```python
from build123d import *

# Parameters (mm, degrees)
PAD_DEPTH       = 5
SKETCH001_R     = 1.75
POCKET_DEPTH    = 5.001
SKETCH002_W     = 36.2
SKETCH002_H     = 26.2
POCKET001_DEPTH = 0.5
SKETCH003_R     = 6
POCKET002_DEPTH = 2.8
POCKET003_DEPTH = 2.8
SKETCH005_W     = 6
SKETCH005_H     = 4.5
POCKET004_DEPTH = 5.001
SKETCH006_W     = 14.7
SKETCH006_H     = 3
POCKET005_DEPTH = 5.001
SKETCH007_W     = 35.7
SKETCH007_H     = 18.1
POCKET006_DEPTH = 4.4
SKETCH008_W     = 1.5
SKETCH008_H     = 8
POCKET007_DEPTH = 3.2
POCKET008_DEPTH = 5.001
SKETCH010_W     = 1
SKETCH010_H     = 2
POCKET009_DEPTH = 5.001


with BuildPart() as part:
    # Sketch → Pad (new body)
    with BuildSketch(Plane.XY):
        Polygon((-25, 14.433757), (-25, -14.433757), (0, -28.867513), (25, -14.433757), (25, 14.433757), (0, 28.867513), align=None)
    extrude(amount=PAD_DEPTH)

    # Sketch001 → Pocket (cut, through all)
    with BuildSketch(Plane.XY.offset(5)):
        with Locations((-10.75, -18.619546)):
            Circle(SKETCH001_R)
        with Locations((10.75, 18.619546)):
            Circle(SKETCH001_R)
    extrude(amount=-POCKET_DEPTH, mode=Mode.SUBTRACT)

    # Sketch002 → Pocket001 (cut)
    with BuildSketch(Plane(origin=(0, 0, 0), x_dir=(1, 0, 0), z_dir=(0, 0, -1))):
        with Locations((-5.9, 0.9)):
            Rectangle(SKETCH002_W, SKETCH002_H)
    extrude(amount=-POCKET001_DEPTH, mode=Mode.SUBTRACT)

    # Sketch003 → Pocket002 (cut)
    with BuildSketch(Plane(origin=(0, 0, 0), x_dir=(1, 0, 0), z_dir=(0, 0, -1))):
        with Locations((0, 21)):
            Circle(SKETCH003_R)
    extrude(amount=-POCKET002_DEPTH, mode=Mode.SUBTRACT)

    # Sketch004 → Pocket003 (cut)
    with BuildSketch(Plane(origin=(0, 0, 0), x_dir=(1, 0, 0), z_dir=(0, 0, -1))):
        Polygon((0.841162, 24.139259), (8.085606, 22.198116), (6.403282, 15.919598), (-0.841162, 17.860741), align=None)
    extrude(amount=-POCKET003_DEPTH, mode=Mode.SUBTRACT)

    # Sketch005 → Pocket004 (cut, through all)
    with BuildSketch(Plane(origin=(0, 0, 0), x_dir=(1, 0, 0), z_dir=(0, 0, -1))):
        with Locations((17.35, 7.05)):
            Rectangle(SKETCH005_W, SKETCH005_H)
    extrude(amount=-POCKET004_DEPTH, mode=Mode.SUBTRACT)

    # Sketch006 → Pocket005 (cut, through all)
    with BuildSketch(Plane(origin=(0, 0, 0), x_dir=(1, 0, 0), z_dir=(0, 0, -1))):
        with Locations((0, -22.4)):
            Rectangle(SKETCH006_W, SKETCH006_H)
    extrude(amount=-POCKET005_DEPTH, mode=Mode.SUBTRACT)

    # Sketch007 → Pocket006 (cut)
    with BuildSketch(Plane.XY.offset(5)):
        with Locations((-5.65, 5.383757)):
            Rectangle(SKETCH007_W, SKETCH007_H)
    extrude(amount=-POCKET006_DEPTH, mode=Mode.SUBTRACT)

    # Sketch008 → Pocket007 (cut)
    with BuildSketch(Plane.XY.offset(5)):
        with Locations((-24.25, 5.383757)):
            Rectangle(SKETCH008_W, SKETCH008_H)
    extrude(amount=-POCKET007_DEPTH, mode=Mode.SUBTRACT)

    # Sketch009 → Pocket008 (cut, through all)
    with BuildSketch(Plane(origin=(0, 0, 0), x_dir=(1, 0, 0), z_dir=(0, 0, -1))):
        Polygon((21.1, 3.15), (24.7, 3.15), (24.7, 2), (25.4, 2), (25.4, -2), (24.7, -2), (24.7, -3.15), (21.1, -3.15), align=None)
    extrude(amount=-POCKET008_DEPTH, mode=Mode.SUBTRACT)

    # Sketch010 → Pocket009 (cut, through all)
    with BuildSketch(Plane(origin=(0, 0, 0), x_dir=(1, 0, 0), z_dir=(0, 0, -1))):
        with Locations((17.55, -11.1)):
            Rectangle(SKETCH010_W, SKETCH010_H)
    extrude(amount=-POCKET009_DEPTH, mode=Mode.SUBTRACT)


solid = part.part
```
Geometry: final body of the model. Coordinates: model frame, mm. A direction names the side the tool comes from. Round coordinates to 2 decimals unless told otherwise and drop trailing zeros. Order: outer loops, then holes, each group sorted by start corner. A loop starts at its lowest first (then second) coordinate and runs counter-clockwise, first axis right, second up. Notation, with made-up numbers: (88.5, 26.25) -> (134.5, 26.25) arc R13 ccw to (134.5, 32.25) -> close; hole circle Ø11 at (-24.5, -29). An arc over 180 degrees is marked (long way). Use one line per item in the form item = value. Start each with the question number.
1. Cut plane B-B (x = -10.75). Return the cut outline in (y, z), then the cut area to 3 significant figures.
2. Cut plane A-A (y = 18). Return the cut outline in (x, z).
3. Cut plane C-C (y = -21). Return the cut outline in (x, z).
4. Cut plane D-D (z = 3.7). Count the separate pieces of the cut face and the enclosed holes in it, then the cut area to 3 significant figures.
5. Line query: probe 1 along X at (y, z) = (11.5, 0.25); probe 2 along Y at (x, z) = (0, 1.3); probe 3 along Y at (x, z) = (-2.5, 4.5). Output: solid intervals per line, ascending.
6. Reachability of faces 4 (the face through (-12.675, -21.55, 2.465)), 5 (the face through (-24, 9.384, 3)), 6 (the face through (-6, -4, 0.5)), 7 (the face through (-6, -3.666, 3)), 8 (the face through (21.1, 0, 2)) from +Z, -Z, +X, -X, +Y, -Y: full face, straight path, thin tool, end or side. Return the list, or none.
7. Draft query along X for faces 1 (the face through (0, -6, 5)), 2 (the face through (-9.94, -20.17, 2.54)), 3 (the face through (25, 8, 2)). Return one class per face: pulls with the +X half, pulls with the -X half, needs draft (parallel to the pull), parting line crosses it, or undercut.
8. Pin query (flat end, axial travel): pin 1 Ø2.5 at (y, z) = (23, 3) entering from +X; pin 2 Ø1.5 at (x, y) = (-19, 10) entering from -Z; pin 3 Ø1.1 at (x, z) = (17.5, 3.5) entering from +Y. Return the tip coordinate at first contact, or that it passes through.
Solution:
q1.outline = (-22.66, 0) -> (-20.37, 0) -> (-20.37, 5) -> (-22.66, 5) -> close; (-16.87, 0) -> (-14, 0) -> (-14, 0.5) -> (12.2, 0.5) -> (12.2, 0) -> (22.66, 0) -> (22.66, 5) -> (14.43, 5) -> (14.43, 0.6) -> (-3.67, 0.6) -> (-3.67, 5) -> (-16.87, 5) -> close
q1.area = 116 mm^2
q2.outline = (-18.82, 0) -> (9.11, 0) -> (9.11, 5) -> (-18.82, 5) -> close; (12.39, 0) -> (18.82, 0) -> (18.82, 5) -> (12.39, 5) -> close
q3.outline = (-13.63, 0) -> (-6, 0) -> (-6, 2.8) -> (7.76, 2.8) -> (7.76, 0) -> (13.63, 0) -> (13.63, 5) -> (-13.63, 5) -> close
q4.separate_pieces = 1
q4.enclosed_holes = 5
q4.area = 1,390 mm^2
q5.probe_1 = -25 to -24, 12.2 to 17.05, 18.05 to 25
q5.probe_2 = -28.87 to -27, -15 to -3.67, 14.43 to 20.9, 23.9 to 28.87
q5.probe_3 = -27.42 to -3.67, 14.43 to 20.9, 23.9 to 27.42
q6.face_4 = +Z, -Z, -X, -Y
q6.face_5 = +Z, -X
q6.face_6 = -Z
q6.face_7 = +Z
q6.face_8 = +Z, -Z
q7.face_1 = needs draft
q7.face_2 = undercut
q7.face_3 = pulls with the +X half
q8.pin_1 = 12.33
q8.pin_2 = 0.5
q8.pin_3 = 19.08
